from build123d import *

# Parameters (mm, degrees)
SKETCH1_W           = 35
SKETCH1_H           = 25
BOSS_EXTRUDE1_DEPTH = 30
SKETCH2_R           = 3.75
CUT_EXTRUDE1_DEPTH  = 5
SKETCH3_R           = 3.75
CUT_EXTRUDE2_DEPTH  = 5


with BuildPart() as part:
    # Sketch1 → Boss-Extrude1 (new body)
    with BuildSketch(Plane(origin=(0, 0, 0), x_dir=(1, 0, 0), z_dir=(0, 1, 0))):
        with Locations((17.5, 12.5)):
            Rectangle(SKETCH1_W, SKETCH1_H)
    extrude(amount=BOSS_EXTRUDE1_DEPTH)

    # Sketch2 → Cut-Extrude1 (cut)
    with BuildSketch(Plane(origin=(35, 0, 0), x_dir=(0, 0, -1), z_dir=(1, 0, 0))):
        with Locations((12.5, 22.5)):
            Circle(SKETCH2_R)
    extrude(amount=-CUT_EXTRUDE1_DEPTH, mode=Mode.SUBTRACT)

    # Sketch3 → Cut-Extrude2 (cut)
    with BuildSketch(Plane.ZY):
        with Locations((-12.5, 22.5)):
            Circle(SKETCH3_R)
    extrude(amount=-CUT_EXTRUDE2_DEPTH, mode=Mode.SUBTRACT)


solid = part.part
For this review, take the finished solid that the model builds, in its own axes (mm). A direction names the side the tool comes from. Round coordinates to 2 decimals unless told otherwise and drop trailing zeros. Order: outer loops, then holes, each group sorted by start corner. A loop starts at its lowest first (then second) coordinate and runs counter-clockwise, first axis right, second up. Notation, with made-up numbers: (-30, -19.5) -> (18, -19.5) arc R21 ccw to (18, -2.5) -> close; hole circle Ø10 at (-9, -5.5). An arc over 180 degrees is marked (long way). Put each result on its own line as item: value.
Q1. Mouldability with a two-part tool opening along Z and no side actions: class faces 1 (the flat face through (35, 15, -12)), 2 (the cylindrical face through (32.53, 18.84, -11.69)), 3 (the flat face through (17, 15, 0)), 4 (the flat face through (17, 15, -25)) as pulls with the +Z half, pulls with the -Z half, needs draft (parallel to the pull), parting line crosses it, or undercut.
Check result:
face 1: needs draft
face 2: undercut
face 3: pulls with the +Z half
face 4: pulls with the -Z half
Q2. Insertion check: pin 1 Ø7 at (y, z) = (22.5, -12.5) entering from -X. The pin has a flat end and moves straight along its axis. Give the tip position at first contact, or say it passes through.
Check result:
pin 1: x = 5
Q3. Add section C-C on z = -12.5. Write out the cut boundary in (x, y), plus the area to 3 significant figures.
Check result:
outline: (0, 0) -> (35, 0) -> (35, 18.75) -> (30, 18.75) -> (30, 26.25) -> (35, 26.25) -> (35, 30) -> (0, 30) -> (0, 26.25) -> (5, 26.25) -> (5, 18.75) -> (0, 18.75) -> close
area: 975 mm2
Q4. Add section B-B on x = 31.5. Write out the cut boundary in (y, z).
Check result:
outline: (0, -25) -> (30, -25) -> (30, 0) -> (0, 0) -> close; hole circle Ø7.5 at (22.5, -12.5)
Q5. For probe 1 along Y at (x, z) = (1.65, -12.5); probe 2 along Y at (x, z) = (3.5, -15), list the stretches that pass through material, from the lowest coordinate up. Write a range as [from, to].
Check result:
probe 1: [0, 18.75], [26.25, 30]
probe 2: [0, 19.7], [25.3, 30]
Q6. Add section A-A on y = 22.5. Write out the cut boundary in (x, z).
Check result:
outline: (0, -25) -> (35, -25) -> (35, -16.25) -> (30, -16.25) -> (30, -8.75) -> (35, -8.75) -> (35, 0) -> (0, 0) -> (0, -8.75) -> (5, -8.75) -> (5, -16.25) -> (0, -16.25) -> close
Q7. Machinability: for faces 5 (the flat face through (17, 0, -13)), 6 (the flat face through (5, 23, -13)), 7 (the flat face through (30, 23, -12)), which of the approach directions +Z, -Z, +X, -X, +Y, -Y give a long, thin tool a straight path to every point of the face, cutting with its end or side? Answer none if there is none.
Check result:
face 5: +Z, -Z, +X, -X, -Y
face 6: -X
face 7: +X
